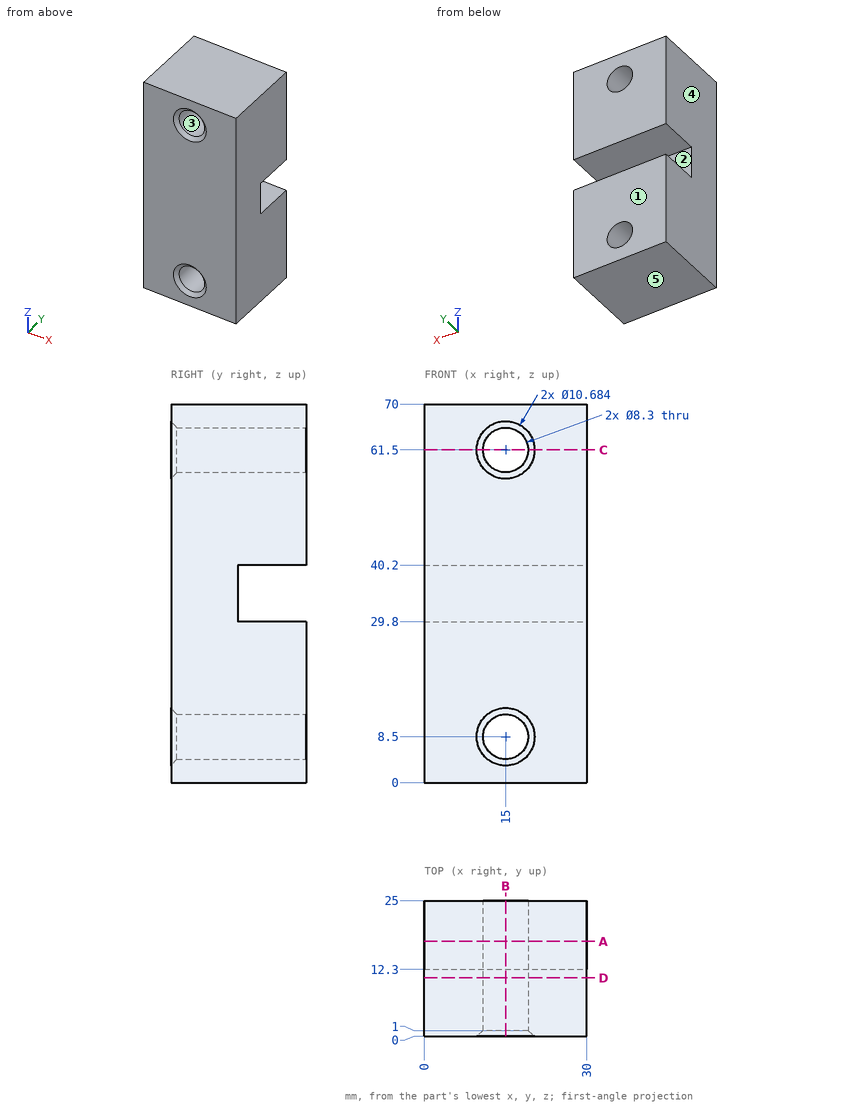
Source: three-view drawing plus pictorial views. Frame: mm from the lowest corner of the part. A direction names the side the tool comes from. Round coordinates to 2 decimals unless told otherwise and drop trailing zeros. Order: outer loops, then holes, each group sorted by start corner. A loop starts at its lowest first (then second) coordinate and runs counter-clockwise, first axis right, second up. Notation, with made-up numbers: (37.5, 27.5) -> (60.5, 27.5) arc R7 cw to (60.5, 34.5) -> close; hole circle Ø9 at (-5, 26). An arc over 180 degrees is marked (long way). Use one line per item in the form item = value. Start each with the question number.
1. Cut plane C-C (z = 61.5). Return the cut outline in (x, y), then the cut area to 3 significant figures.
2. Line query: probe 1 along Z at (x, y) = (15, 7.5); probe 2 along X at (y, z) = (10.75, 61.5); probe 3 along Z at (x, y) = (12.25, 8). Output: solid intervals per line, ascending.
3. Pin query (flat end, axial travel): pin 1 Ø5 at (x, z) = (15, 61.5) entering from +Y. Return the tip coordinate at first contact, or that it passes through.
4. Cut plane A-A (y = 17.5). Return the cut outline in (x, z), then the cut area to 3 significant figures.
5. Cut plane D-D (y = 10.75). Return the cut outline in (x, z).
6. Reachability of the marked faces 1 and 2 from +Z, -Z, +X, -X, +Y, -Y: full face, straight path, thin tool, end or side. Return the list, or none.
7. Cut plane B-B (x = 15). Return the cut outline in (y, z), then the cut area to 3 significant figures.
8. Draft query along Z for the marked faces 3, 4 and 5. Return one class per face: pulls with the +Z half, pulls with the -Z half, needs draft (parallel to the pull), parting line crosses it, or undercut.
Solution:
q1.outline = (0, 0) -> (9.66, 0) -> (10.85, 1) -> (10.85, 25) -> (0, 25) -> close; (19.15, 1) -> (20.34, 0) -> (30, 0) -> (30, 25) -> (19.15, 25) -> close
q1.area = 541 mm^2
q2.probe_1 = 0 to 4.35, 12.65 to 57.35, 65.65 to 70
q2.probe_2 = 0 to 10.85, 19.15 to 30
q2.probe_3 = 0 to 5.39, 11.61 to 58.39, 64.61 to 70
q3.pin_1 = through
q4.outline = (0, 0) -> (30, 0) -> (30, 29.8) -> (0, 29.8) -> close; (0, 40.2) -> (30, 40.2) -> (30, 70) -> (0, 70) -> close; hole circle Ø8.3 at (15, 8.5); hole circle Ø8.3 at (15, 61.5)
q4.area = 1,680 mm^2
q5.outline = (0, 0) -> (30, 0) -> (30, 70) -> (0, 70) -> close; hole circle Ø8.3 at (15, 8.5); hole circle Ø8.3 at (15, 61.5)
q6.face_1 = +Z, -Z, +X, -X, +Y
q6.face_2 = +X, -X, +Y
q7.outline = (0, 0) -> (25, 0) -> (25, 4.35) -> (1, 4.35) -> (0, 3.16) -> close; (0, 13.84) -> (1, 12.65) -> (25, 12.65) -> (25, 29.8) -> (12.3, 29.8) -> (12.3, 40.2) -> (25, 40.2) -> (25, 57.35) -> (1, 57.35) -> (0, 56.16) -> close; (0, 66.84) -> (1, 65.65) -> (25, 65.65) -> (25, 70) -> (0, 70) -> close
q7.area = 1,200 mm^2
q8.face_3 = undercut
q8.face_4 = needs draft
q8.face_5 = pulls with the -Z half
